```python
from build123d import *

# Parameters (mm, degrees)
SKETCH1_R               = 12.5
SKETCH1_R_2             = 8.5
BOSS_EXTRUDE1_DEPTH     = 400
CUT_EXTRUDE1_DEPTH      = 401.390434451
CUT_EXTRUDE1_DEPTH_BACK = 401.390434451
SKETCH2_R               = 1.5
CUT_EXTRUDE2_DEPTH      = 401.390434558
CUT_EXTRUDE2_DEPTH_BACK = 401.390434558
SKETCH3_R               = 1.5
CUT_EXTRUDE3_DEPTH      = 401.390434559
CUT_EXTRUDE3_DEPTH_BACK = 110
SKETCH4_R               = 16.409503563


with BuildPart() as part:
    # Sketch1 → Boss-Extrude1 (new body)
    with BuildSketch(Plane.XY):
        Circle(SKETCH1_R)
        Circle(SKETCH1_R_2, mode=Mode.SUBTRACT)
    extrude(amount=BOSS_EXTRUDE1_DEPTH)

    # Sketch2 → Cut-Extrude1 (cut, two sides: drawn at the far end of the back side and taken through both)
    with BuildSketch(Plane(origin=(0, 0, 0), x_dir=(1, 0, 0), z_dir=(0, 1, 0)).offset(-CUT_EXTRUDE1_DEPTH_BACK)):
        with Locations(Location((0, -370, 0), (0, 0, 270))):
            Circle(SKETCH2_R)
        with Locations(Location((0, -280, 0), (0, 0, 270))):
            Circle(SKETCH2_R)
    extrude(amount=CUT_EXTRUDE1_DEPTH + CUT_EXTRUDE1_DEPTH_BACK, mode=Mode.SUBTRACT)

    # Sketch3 → Cut-Extrude2 (cut, two sides: drawn at the far end of the back side and taken through both)
    with BuildSketch(Plane(origin=(0, 0, 0), x_dir=(0, 0, -1), z_dir=(1, 0, 0)).offset(-CUT_EXTRUDE2_DEPTH_BACK)):
        with Locations((-121, 0)):
            Circle(SKETCH3_R)
        with Locations((-140, 0)):
            Circle(SKETCH3_R)
    extrude(amount=CUT_EXTRUDE2_DEPTH + CUT_EXTRUDE2_DEPTH_BACK, mode=Mode.SUBTRACT)

    # Sketch4 → Cut-Extrude3 (cut, two sides: drawn at the far end of the back side and taken through both)
    with BuildSketch(Plane(origin=(0, 0, 0), x_dir=(-1, 0, 0), z_dir=(0, 0, -1)).offset(-CUT_EXTRUDE3_DEPTH_BACK)):
        Circle(SKETCH4_R)
    extrude(amount=CUT_EXTRUDE3_DEPTH + CUT_EXTRUDE3_DEPTH_BACK, mode=Mode.SUBTRACT)


solid = part.part
```
Could you check a few things on this model? Use its own coordinates, in mm. Coordinates: 2 decimals unless noted, no trailing zeros. Write each loop counter-clockwise with the first axis right and the second up, starting at its lowest first coordinate (ties: lowest second). Pieces come first, ordered by that corner, then holes. Notation, with made-up numbers: (-1, -5.75) - (7, -5.75) arc R36 cw to (7, 33.25) - close; hole circle Ø9 at (65.5, 28). An arc over 180 degrees is marked (long way). Use a Markdown table: item, result.
Q1. Thinking about a two-plate mould opening in X: for faces 1 (the cylindrical face through (11.923, 3.755, 252.97)), 2 (the cylindrical face through (4.57, 7.167, 252.97)), 3 (the flat face through (-3, -8.2, 400)), which applies, +X half, -X half, draft (parallel to the pull), parting line (faces both ways), or undercut?
Geometry check:
| item | result |
|---|---|
| face 1 | parting line |
| face 2 | undercut |
| face 3 | draft |
Q2. Imagine slicing it at A-A (y = -5.75). List the corners of the cut face in (x, z) for me.
Geometry check:
| item | result |
|---|---|
| outline | (-11.1, 110) - (-6.26, 110) - (-6.26, 400) - (-11.1, 400) - close; (6.26, 110) - (11.1, 110) - (11.1, 400) - (6.26, 400) - close |
Q3. Please list where these lines run through material, in increasing order: L1, parallel to Z at x = 0, y = 10.4; L2, parallel to Z at x = 10.7, y = 0; L3, parallel to X at y = -0.5, z = 305.5.
Geometry check:
| item | result |
|---|---|
| L1 | z = 110 to 278.5, 281.5 to 368.5, 371.5 to 400 |
| L2 | z = 110 to 119.5, 122.5 to 138.5, 141.5 to 400 |
| L3 | x = -12.49 to -8.49, 8.49 to 12.49 |
Q4. Imagine slicing it at C-C (z = 365.5). List the corners of the cut face in (x, y) for me.
Geometry check:
| item | result |
|---|---|
| outline | circle Ø25 at (0, 0); hole circle Ø17 at (0, 0) |
Q5. Imagine slicing it at B-B (x = 4.75). List the corners of the cut face in (y, z) for me.
Geometry check:
| item | result |
|---|---|
| outline | (-11.56, 110) - (-7.05, 110) - (-7.05, 400) - (-11.56, 400) - close; (7.05, 110) - (11.56, 110) - (11.56, 400) - (7.05, 400) - close |
Q6. I'm going to push flat-ended pins straight in: pin 1 Ø2.5 at (x, z) = (0, 280) entering from -Y; pin 2 Ø4 at (x, z) = (-6.5, 285.5) entering from -Y; pin 3 Ø3 at (x, z) = (4.5, 151.5) entering from -Y; pin 4 Ø1.5 at (y, z) = (8, 294.5) entering from -X. Where does each tip first touch, or does it pass through?
Geometry check:
| item | result |
|---|---|
| pin 1 | passes through |
| pin 2 | stops at y = -11.66 |
| pin 3 | stops at y = -12.13 |
| pin 4 | stops at x = -10.18 |
